```python
from build123d import *

# Parameters (mm, degrees)
SKETCH1_R           = 127
BOSS_EXTRUDE1_DEPTH = 25.4
BOSS_EXTRUDE2_DEPTH = 6.35


with BuildPart() as part:
    # Sketch1 → Boss-Extrude1 (new body)
    with BuildSketch(Plane(origin=(0, 0, 0), x_dir=(1, 0, 0), z_dir=(0, 1, 0))):
        with Locations(Location((0, 0, 0), (0, 0, 270))):
            Circle(SKETCH1_R)
    extrude(amount=BOSS_EXTRUDE1_DEPTH)

    # Sketch2 → Boss-Extrude2 (add)
    with BuildSketch(Plane(origin=(0, 25.4, 0), x_dir=(1, 0, 0), z_dir=(0, 1, 0))):
        with BuildLine():
            Line((-126.592947671, 10.16), (-17.597636205, 10.16))
            Line((-17.597636205, 10.16), (-72.095291938, 104.552708623))
            ThreePointArc((-72.095291938, 104.552708623), (-74.182318509, 103.082411791), (-76.239369275, 101.570461122))
            Line((-76.239369275, 101.570461122), (-26.396454307, 15.24))
            Line((-26.396454307, 15.24), (-126.082284243, 15.24))
            ThreePointArc((-126.082284243, 15.24), (-126.363146549, 12.702566445), (-126.592947671, 10.16))
        make_face()
        with BuildLine():
            Line((-126.082284243, -15.24), (-26.396454307, -15.24))
            Line((-26.396454307, -15.24), (-76.239369275, -101.570461122))
            ThreePointArc((-76.239369275, -101.570461122), (-74.182318509, -103.082411791), (-72.095291938, -104.552708623))
            Line((-72.095291938, -104.552708623), (-17.597636205, -10.16))
            Line((-17.597636205, -10.16), (-126.592947671, -10.16))
            ThreePointArc((-126.592947671, -10.16), (-126.363146549, -12.702566445), (-126.082284243, -15.24))
        make_face()
        with BuildLine():
            Line((54.497655733, -114.712708623), (0, -20.32))
            Line((0, -20.32), (-54.497655733, -114.712708623))
            ThreePointArc((-54.497655733, -114.712708623), (-52.18082804, -115.784978236), (-49.842914968, -116.810461122))
            Line((-49.842914968, -116.810461122), (0, -30.48))
            Line((0, -30.48), (49.842914968, -116.810461122))
            ThreePointArc((49.842914968, -116.810461122), (52.18082804, -115.784978236), (54.497655733, -114.712708623))
        make_face()
        with BuildLine():
            Line((76.239369275, -101.570461122), (26.396454307, -15.24))
            Line((26.396454307, -15.24), (126.082284243, -15.24))
            ThreePointArc((126.082284243, -15.24), (126.363146549, -12.702566445), (126.592947671, -10.16))
            Line((126.592947671, -10.16), (17.597636205, -10.16))
            Line((17.597636205, -10.16), (72.095291938, -104.552708623))
            ThreePointArc((72.095291938, -104.552708623), (74.182318509, -103.082411791), (76.239369275, -101.570461122))
        make_face()
        with BuildLine():
            Line((72.095291938, 104.552708623), (17.597636205, 10.16))
            Line((17.597636205, 10.16), (126.592947671, 10.16))
            ThreePointArc((126.592947671, 10.16), (126.363146549, 12.702566445), (126.082284243, 15.24))
            Line((126.082284243, 15.24), (26.396454307, 15.24))
            Line((26.396454307, 15.24), (76.239369275, 101.570461122))
            ThreePointArc((76.239369275, 101.570461122), (74.182318509, 103.082411791), (72.095291938, 104.552708623))
        make_face()
        with BuildLine():
            Line((49.842914968, 116.810461122), (0, 30.48))
            Line((0, 30.48), (-49.842914968, 116.810461122))
            ThreePointArc((-49.842914968, 116.810461122), (-52.18082804, 115.784978236), (-54.497655733, 114.712708623))
            Line((-54.497655733, 114.712708623), (0, 20.32))
            Line((0, 20.32), (54.497655733, 114.712708623))
            ThreePointArc((54.497655733, 114.712708623), (52.18082804, 115.784978236), (49.842914968, 116.810461122))
        make_face()
    extrude(amount=BOSS_EXTRUDE2_DEPTH)


solid = part.part
```
Build history of the part. All positions in model axes, mm. A direction names the side the tool comes from. Give positions to 0.01 mm unless a question says otherwise; leave off trailing zeros. Loops run counter-clockwise (first coordinate to the right, second up) from the corner with the lowest first, then second, coordinate; pieces in that order, holes last.
1) Two-plate mould, pull along X, no slides. Class faces 1 (the face through (45.23, 28.53, -58.02)), 2 (the face through (50.97, 28.53, -57.8)), 3 (the face through (73, 29, 10.16)), 4 (the face through (1, 25.4, -9)): released by +X, released by -X, zero draft, split by the parting line, or undercut.
Values follow:
face 1: undercut
face 2: released by +X
face 3: zero draft
face 4: undercut
2) Band-saw the part on B-B on x = -36. List the corners of the cut face in (y, z).
Values follow:
outline: (0, -121.79) - (25.4, -121.79) - (25.4, -92.83) - (31.75, -92.83) - (31.75, -82.67) - (25.4, -82.67) - (25.4, -42.03) - (31.75, -42.03) - (31.75, -31.87) - (25.4, -31.87) - (25.4, -15.24) - (31.75, -15.24) - (31.75, -10.16) - (25.4, -10.16) - (25.4, 10.16) - (31.75, 10.16) - (31.75, 15.24) - (25.4, 15.24) - (25.4, 31.87) - (31.75, 31.87) - (31.75, 42.03) - (25.4, 42.03) - (25.4, 82.67) - (31.75, 82.67) - (31.75, 92.83) - (25.4, 92.83) - (25.4, 121.79) - (0, 121.79) - close
3) Band-saw the part on D-D on z = 73. List the corners of the cut face in (x, y), then the cut area to 3 significant figures.
Values follow:
outline: (-103.92, 0) - (103.92, 0) - (103.92, 25.4) - (59.74, 25.4) - (59.74, 31.75) - (53.88, 31.75) - (53.88, 25.4) - (30.41, 25.4) - (30.41, 31.75) - (24.55, 31.75) - (24.55, 25.4) - (-24.55, 25.4) - (-24.55, 31.75) - (-30.41, 31.75) - (-30.41, 25.4) - (-53.88, 25.4) - (-53.88, 31.75) - (-59.74, 31.75) - (-59.74, 25.4) - (-103.92, 25.4) - close
area: 5,430 mm2
4) 3-axis set-ups, long thin cutter, end or side, ignore diameter. For faces 5 (the face through (27.63, 28.53, 68.18)), 6 (the face through (-24.57, 28.53, -73.04)), 7 (the face through (-76, 25.4, -49)), 8 (the face through (71, 29, -10.16)), 9 (the face through (77, 25.4, 48)): which of +Z, -Z, +X, -X, +Y, -Y reach the whole face in a straight line?
Values follow:
face 5: +Y
face 6: -Z, +Y
face 7: -X, +Y
face 8: +X, -X, +Y
face 9: +X, +Y
5) Probe line 1 along Z through (x, y) = (117, 27); line 2 along X through (y, z) = (30, -98.5); line 3 along Y through (x, z) = (-12, -19). List the from-to ranges inside material, lowest first.
Values follow:
line 1: z = -15.24 to -10.16, 10.16 to 15.24
line 2: x = -74.47 to -68.6, -45.14 to -39.27, 39.27 to 45.14, 68.6 to 74.47
line 3: y = 0 to 25.4
6) Band-saw the part on A-A on z = -79. List the corners of the cut face in (x, y), then the cut area to 3 significant figures.
Values follow:
outline: (-99.44, 0) - (99.44, 0) - (99.44, 25.4) - (63.21, 25.4) - (63.21, 31.75) - (57.34, 31.75) - (57.34, 25.4) - (33.88, 25.4) - (33.88, 31.75) - (28.01, 31.75) - (28.01, 25.4) - (-28.01, 25.4) - (-28.01, 31.75) - (-33.88, 31.75) - (-33.88, 25.4) - (-57.34, 25.4) - (-57.34, 31.75) - (-63.21, 31.75) - (-63.21, 25.4) - (-99.44, 25.4) - close
area: 5,200 mm2
7) Drop flat-ended pins along their axis: P1, Ø8, axis at y = 11, z = 60, coming from the -X side; P2, Ø12, axis at x = -93, y = 23.5, coming from the +Z side; P3, Ø1.9, axis at x = -66, y = 27.5, coming from the +Z side. Give the stop position or say it passes through.
Values follow:
P1: stops at x = -113.99
P2: stops at z = 92.52
P3: stops at z = 95.64
8) Band-saw the part on C-C on y = 5.5. List the corners of the cut face in (x, z).
Values follow:
outline: circle Ø254 at (0, 0)
